```python
from build123d import *

# Parameters (mm, degrees)
SKETCH1_W                  = 275
SKETCH1_H                  = 33
BOSS_EXTRUDE1_DEPTH        = 12
CUT_EXTRUDE1_REACH         = 141.005
SKETCH2_R                  = 10
SKETCH2_R_2                = 2.5
SKETCH3_W                  = 366
SKETCH3_H                  = 117
BOSS_EXTRUDE2_DEPTH        = 12
CUT_EXTRUDE2_REACH         = 308.55
SKETCH4_R                  = 2.5
CUT_EXTRUDE3_REACH         = 343.869
SKETCH5_W                  = 14
SKETCH5_H                  = 6
FILLET1_R                  = 2
FILLET1_OF_MIRROR2_R       = 2
CHAMFER1_SIZE              = 10
CUT_EXTRUDE6_REACH         = 343.869
SKETCH8_W                  = 12
SKETCH8_H                  = 42
CHAMFER2_SIZE              = 10
F_6_0_6_DIAMETER_HOLE1_D   = 6
F_10_0_10_DIAMETER_HOLE1_D = 10
F_6_0_6_DIAMETER_HOLE4_D   = 6


with BuildPart() as part:
    # Sketch1 → Boss-Extrude1 (new body)
    with BuildSketch(Plane.XY):
        Rectangle(SKETCH1_W, SKETCH1_H)
    extrude(amount=BOSS_EXTRUDE1_DEPTH)

    # Sketch2 → Cut-Extrude1 (cut, up to next)
    with BuildSketch(Plane.XY.offset(12), mode=Mode.PRIVATE) as cut_extrude1_sk1:
        with Locations((0, 1)):
            Circle(SKETCH2_R)
    cut_extrude1_tool1 = extrude(cut_extrude1_sk1.sketch, amount=-CUT_EXTRUDE1_REACH, mode=Mode.PRIVATE) & part.part
    # Sketch2 → Cut-Extrude1 (cut, up to next)
    with BuildSketch(Plane.XY.offset(12), mode=Mode.PRIVATE) as cut_extrude1_sk2:
        with Locations((-15, 1)):
            Circle(SKETCH2_R_2)
    cut_extrude1_tool2 = extrude(cut_extrude1_sk2.sketch, amount=-CUT_EXTRUDE1_REACH, mode=Mode.PRIVATE) & part.part
    # Sketch2 → Cut-Extrude1 (cut, up to next)
    with BuildSketch(Plane.XY.offset(12), mode=Mode.PRIVATE) as cut_extrude1_sk3:
        with Locations((15, 1)):
            Circle(SKETCH2_R_2)
    cut_extrude1_tool3 = extrude(cut_extrude1_sk3.sketch, amount=-CUT_EXTRUDE1_REACH, mode=Mode.PRIVATE) & part.part
    add(cut_extrude1_tool1.solids().sort_by_distance((0, 1, 12))[0], mode=Mode.SUBTRACT)
    add(cut_extrude1_tool2.solids().sort_by_distance((-15, 1, 12))[0], mode=Mode.SUBTRACT)
    add(cut_extrude1_tool3.solids().sort_by_distance((15, 1, 12))[0], mode=Mode.SUBTRACT)

    # Sketch3 → Boss-Extrude2 (add)
    with BuildSketch(Plane.XY.offset(12)):
        Polygon((-210, 16.5), (210, 16.5), (210, 46.5), (210, 269.5), (-210, 269.5), (-210, 46.5), align=None)
        with Locations((0, 105)):
            Rectangle(SKETCH3_W, SKETCH3_H, mode=Mode.SUBTRACT)
    extrude(amount=-BOSS_EXTRUDE2_DEPTH)

    # Sketch4 → Cut-Extrude2 (cut, up to next)
    with BuildSketch(Plane(origin=(0, 46.5, 0), x_dir=(1, 0, 0), z_dir=(0, 1, 0)), mode=Mode.PRIVATE) as cut_extrude2_sk1:
        with Locations(Location((-144, -6, 0), (0, 0, 270))):
            Circle(SKETCH4_R)
    cut_extrude2_tool1 = extrude(cut_extrude2_sk1.sketch, amount=-CUT_EXTRUDE2_REACH, mode=Mode.PRIVATE) & part.part
    # Sketch4 → Cut-Extrude2 (cut, up to next)
    with BuildSketch(Plane(origin=(0, 46.5, 0), x_dir=(1, 0, 0), z_dir=(0, 1, 0)), mode=Mode.PRIVATE) as cut_extrude2_sk2:
        with Locations(Location((-176, -6, 0), (0, 0, 270))):
            Circle(SKETCH4_R)
    cut_extrude2_tool2 = extrude(cut_extrude2_sk2.sketch, amount=-CUT_EXTRUDE2_REACH, mode=Mode.PRIVATE) & part.part
    cut_extrude2_1 = cut_extrude2_tool1.solids().sort_by_distance((-144, 46.5, 6))[0]
    add(cut_extrude2_1, mode=Mode.SUBTRACT)
    cut_extrude2_2 = cut_extrude2_tool2.solids().sort_by_distance((-176, 46.5, 6))[0]
    add(cut_extrude2_2, mode=Mode.SUBTRACT)
    cut_extrude2 = cut_extrude2_1 + cut_extrude2_2  # Cut-Extrude2 as one shape, for the pattern or mirror that repeats it

    # Mirror1: Cut-Extrude2 across plane
    add(cut_extrude2.mirror(Plane(origin=(0, 0, 0), x_dir=(0, 0, 1), z_dir=(1, 0, 0))), mode=Mode.SUBTRACT)

    # Sketch5 → Cut-Extrude3 (cut, up to next)
    with BuildSketch(Plane.XY.offset(12), mode=Mode.PRIVATE) as cut_extrude3_sk1:
        with Locations((-176, 43.5)):
            Rectangle(SKETCH5_W, SKETCH5_H)
    cut_extrude3_tool1 = extrude(cut_extrude3_sk1.sketch, amount=-CUT_EXTRUDE3_REACH, mode=Mode.PRIVATE) & part.part
    # Sketch5 → Cut-Extrude3 (cut, up to next)
    with BuildSketch(Plane.XY.offset(12), mode=Mode.PRIVATE) as cut_extrude3_sk2:
        with Locations((-144, 43.5)):
            Rectangle(SKETCH5_W, SKETCH5_H)
    cut_extrude3_tool2 = extrude(cut_extrude3_sk2.sketch, amount=-CUT_EXTRUDE3_REACH, mode=Mode.PRIVATE) & part.part
    cut_extrude3_1 = cut_extrude3_tool1.solids().sort_by_distance((-176, 43.5, 12))[0]
    add(cut_extrude3_1, mode=Mode.SUBTRACT)
    cut_extrude3_2 = cut_extrude3_tool2.solids().sort_by_distance((-144, 43.5, 12))[0]
    add(cut_extrude3_2, mode=Mode.SUBTRACT)
    cut_extrude3 = cut_extrude3_1 + cut_extrude3_2  # Cut-Extrude3 as one shape, for the pattern or mirror that repeats it

    # Fillet1
    fillet1_edges = [part.edges().sort_by_distance(p)[0] for p in [
        (-169, 40.5, 6),
        (-183, 40.5, 6),
        (-137, 40.5, 6),
        (-151, 40.5, 6),
    ]]
    fillet(fillet1_edges, radius=FILLET1_R)

    # Mirror2: Cut-Extrude3 across plane
    add(cut_extrude3.mirror(Plane(origin=(0, 0, 0), x_dir=(0, 0, 1), z_dir=(1, 0, 0))), mode=Mode.SUBTRACT)

    # Fillet1 of Mirror2
    fillet1_of_mirror2_edges = [part.edges().sort_by_distance(p)[0] for p in [
        (169, 40.5, 6),
        (183, 40.5, 6),
        (137, 40.5, 6),
        (151, 40.5, 6),
    ]]
    fillet(fillet1_of_mirror2_edges, radius=FILLET1_OF_MIRROR2_R)

    # Chamfer1
    chamfer1_edges = [part.edges().sort_by_distance(p)[0] for p in [
        (210, 16.5, 6),
        (-210, 16.5, 6),
    ]]
    chamfer(chamfer1_edges, length=CHAMFER1_SIZE)

    # Sketch8 → Cut-Extrude6 (cut, up to next)
    with BuildSketch(Plane.XY.offset(12), mode=Mode.PRIVATE) as cut_extrude6_sk1:
        with Locations((-194, 248.5)):
            Rectangle(SKETCH8_W, SKETCH8_H)
    cut_extrude6_tool1 = extrude(cut_extrude6_sk1.sketch, amount=-CUT_EXTRUDE6_REACH, mode=Mode.PRIVATE) & part.part
    # Sketch8 → Cut-Extrude6 (cut, up to next)
    with BuildSketch(Plane.XY.offset(12), mode=Mode.PRIVATE) as cut_extrude6_sk2:
        with Locations((194, 248.5)):
            Rectangle(SKETCH8_W, SKETCH8_H)
    cut_extrude6_tool2 = extrude(cut_extrude6_sk2.sketch, amount=-CUT_EXTRUDE6_REACH, mode=Mode.PRIVATE) & part.part
    add(cut_extrude6_tool1.solids().sort_by_distance((-194, 248.5, 12))[0], mode=Mode.SUBTRACT)
    add(cut_extrude6_tool2.solids().sort_by_distance((194, 248.5, 12))[0], mode=Mode.SUBTRACT)

    # Chamfer2
    chamfer2_edges = [part.edges().sort_by_distance(p)[0] for p in [
        (210, 269.5, 6),
        (-210, 269.5, 6),
    ]]
    chamfer(chamfer2_edges, length=CHAMFER2_SIZE - 0.0001)  # a hair under: the kernel refuses the full size

    # Ø6.0 (6) Diameter Hole1 (through all)
    with Locations(Plane(origin=(0, 0, 0), x_dir=(-1, 0, 0), z_dir=(0, 0, -1))):
        with Locations((195, 131.5), (195, 40.5)):
            f_6_0_6_diameter_hole1 = Hole(F_6_0_6_DIAMETER_HOLE1_D / 2)

    # Ø10.0 (10) Diameter Hole1 (through all)
    with Locations(Plane(origin=(0, 0, 0), x_dir=(-1, 0, 0), z_dir=(0, 0, -1))):
        with Locations((176, 245.5)):
            f_10_0_10_diameter_hole1 = Hole(F_10_0_10_DIAMETER_HOLE1_D / 2)

    # Sketch13 → Ø6.0 (6) Diameter Hole2 (revolve, cut)
    with BuildSketch(Plane(origin=(-188, 245.5, 6), x_dir=(0, 0, 1), z_dir=(0, 1, 0))):
        Polygon((0, 0), (0, 21.802581857), (3, 20), (3, 0), align=None)
    f_6_0_6_diameter_hole2 = revolve(axis=Axis((-194.35, 245.5, 6), (1, 0, 0)), mode=Mode.SUBTRACT)

    # Sketch15 → Ø6.0 (6) Diameter Hole3 (revolve, cut)
    with BuildSketch(Plane(origin=(-210, 245.5, 6), x_dir=(0, 0, 1), z_dir=(0, 1, 0))):
        Polygon((0, 0), (0, 21.802581857), (3, 20), (3, 0), align=None)
    f_6_0_6_diameter_hole3 = revolve(axis=Axis((-216.35, 245.5, 6), (1, 0, 0)), mode=Mode.SUBTRACT)

    # Mirror3: Ø6.0 (6) Diameter Hole1, Ø10.0 (10) Diameter Hole1, Ø6.0 (6) Diameter Hole2, Ø6.0 (6) Diameter Hole3 across plane
    add(f_6_0_6_diameter_hole1.mirror(Plane(origin=(0, 0, 0), x_dir=(0, 0, 1), z_dir=(1, 0, 0))), mode=Mode.SUBTRACT)
    add(f_10_0_10_diameter_hole1.mirror(Plane(origin=(0, 0, 0), x_dir=(0, 0, 1), z_dir=(1, 0, 0))), mode=Mode.SUBTRACT)
    add(f_6_0_6_diameter_hole2.mirror(Plane(origin=(0, 0, 0), x_dir=(0, 0, 1), z_dir=(1, 0, 0))), mode=Mode.SUBTRACT)
    add(f_6_0_6_diameter_hole3.mirror(Plane(origin=(0, 0, 0), x_dir=(0, 0, 1), z_dir=(1, 0, 0))), mode=Mode.SUBTRACT)

    # Ø6.0 (6) Diameter Hole4 (through all)
    with Locations(Plane(origin=(0, 0, 0), x_dir=(-1, 0, 0), z_dir=(0, 0, -1))):
        with Locations((-97.5, 13.5), (-40, 13.5), (40, 13.5), (97.5, 13.5)):
            Hole(F_6_0_6_DIAMETER_HOLE4_D / 2)


solid = part.part
```
The model under review builds one solid part; all positions refer to its coordinate system, in mm. A direction names the side the tool comes from. Coordinates: 2 decimals unless noted, no trailing zeros. Write each loop counter-clockwise with the first axis right and the second up, starting at its lowest first coordinate (ties: lowest second). Pieces come first, ordered by that corner, then holes.
1) We need section B-B on y = 147.5. State the section outline as (x, z) points, then the cut area to 3 significant figures.
2) Clearance check with flat-ended pins moving along their axes: pin 1 Ø5.5 at (x, y) = (40, 13.5) entering from +Z; pin 2 Ø3.5 at (x, z) = (180, 9) entering from -Y. State where each tip first meets the part, or that it passes through.
3) To check wall thickness, follow probe 1 along X at (y, z) = (131.5, 4.5); probe 2 along Y at (x, z) = (-15, 3.5); probe 3 along X at (y, z) = (116, 10.5). State the ranges of each line that lie inside material, in increasing order.
4) We need section A-A on x = -23.5. State the section outline as (y, z) points, then the cut area to 3 significant figures.
5) Machinability: for faces 5 (the face through (-3, 192, 0)), 6 (the face through (188, 248, 9)), 7 (the face through (168, 16.5, 6)), 8 (the face through (146.3, 40.5, 7.4)), which of the approach directions +Z, -Z, +X, -X, +Y, -Y give a long, thin tool a straight path to every point of the face, cutting with its end or side? Answer none if there is none.
6) The part is to be moulded in two halves that separate along X. For faces 1 (the face through (-3, 192, 12)), 2 (the face through (137.5, 0, 6)), 3 (the face through (-204.9, 264.6, 6.1)), 4 (the face through (-2, 46.5, 6)), say which applies: pulls with the +X half, pulls with the -X half, needs draft (parallel to the pull), parting line crosses it, or undercut.
Answer list:
1. outline: (-210, 0) - (-183, 0) - (-183, 12) - (-210, 12) - close; (183, 0) - (210, 0) - (210, 12) - (183, 12) - close
1. area: 648 mm2
2. pin 1: passes through
2. pin 2: stops at y = 16.5
3. probe 1: x = -210 to -198, -192 to -183, 183 to 192, 198 to 210
3. probe 2: y = -16.5 to -1.5, 3.5 to 46.5, 163.5 to 269.5
3. probe 3: x = -210 to -183, 183 to 210
4. outline: (-16.5, 0) - (46.5, 0) - (46.5, 12) - (-16.5, 12) - close; (163.5, 0) - (269.5, 0) - (269.5, 12) - (163.5, 12) - close
4. area: 2,030 mm2
5. face 5: -Z, +X, -X, +Y, -Y
5. face 6: +Z, -Z, +Y
5. face 7: +Z, -Z, +X, -Y
5. face 8: +Z, -Z
6. face 1: needs draft
6. face 2: pulls with the +X half
6. face 3: pulls with the -X half
6. face 4: undercut
